from build123d import *

# Parameters (mm, degrees)
CROQUIS1_W              = 8
CROQUIS1_H              = 8
CROQUIS1_R              = 2.5
SALIENTE_EXTRUIR4_DEPTH = 150


with BuildPart() as part:
    # Croquis1 → Saliente-Extruir4 (new body)
    with BuildSketch(Plane.XY):
        with BuildLine():
            Line((-3, 8.7), (-3, 10))
            Line((-3, 10), (-9, 10))
            ThreePointArc((-9, 10), (-9.707106781, 9.707106781), (-10, 9))
            Line((-10, 9), (-10, 3))
            Line((-10, 3), (-8.7, 3))
            Line((-8.7, 3), (-8.7, 6))
            Line((-8.7, 6), (-4, 3.25))
            Line((-4, 3.25), (-4, 4))
            Line((-4, 4), (-3.25, 4))
            Line((-3.25, 4), (-6, 8.7))
            Line((-6, 8.7), (-3, 8.7))
        make_face()
        with BuildLine():
            Line((9, 10), (3, 10))
            Line((3, 10), (3, 8.7))
            Line((3, 8.7), (6, 8.7))
            Line((6, 8.7), (3.25, 4))
            Line((3.25, 4), (4, 4))
            Line((4, 4), (4, 3.25))
            Line((4, 3.25), (8.7, 6))
            Line((8.7, 6), (8.7, 3))
            Line((8.7, 3), (10, 3))
            Line((10, 3), (10, 9))
            ThreePointArc((10, 9), (9.707106781, 9.707106781), (9, 10))
        make_face()
        with BuildLine():
            Line((10, -9), (10, -3))
            Line((10, -3), (8.7, -3))
            Line((8.7, -3), (8.7, -6))
            Line((8.7, -6), (4, -3.25))
            Line((4, -3.25), (4, -4))
            Line((4, -4), (3.25, -4))
            Line((3.25, -4), (6.25, -8.7))
            Line((6.25, -8.7), (3, -8.7))
            Line((3, -8.7), (3, -10))
            Line((3, -10), (9, -10))
            ThreePointArc((9, -10), (9.707106781, -9.707106781), (10, -9))
        make_face()
        with BuildLine():
            Line((-8.7, -3), (-10, -3))
            Line((-10, -3), (-10, -9))
            ThreePointArc((-10, -9), (-9.707106781, -9.707106781), (-9, -10))
            Line((-9, -10), (-3, -10))
            Line((-3, -10), (-3, -8.7))
            Line((-3, -8.7), (-5.75, -8.7))
            Line((-5.75, -8.7), (-3.25, -4))
            Line((-3.25, -4), (-4, -4))
            Line((-4, -4), (-4, -3.25))
            Line((-4, -3.25), (-8.7, -6))
            Line((-8.7, -6), (-8.7, -3))
        make_face()
        Rectangle(CROQUIS1_W, CROQUIS1_H)
        Circle(CROQUIS1_R, mode=Mode.SUBTRACT)
    extrude(amount=SALIENTE_EXTRUIR4_DEPTH)


solid = part.part
Work out the finished part from the listing and answer in its coordinate system (mm). A direction names the side the tool comes from. Round coordinates to 2 decimals unless told otherwise and drop trailing zeros. Write each loop counter-clockwise with the first axis right and the second up, starting at its lowest first coordinate (ties: lowest second). Pieces come first, ordered by that corner, then holes.
1) A cutting plane is placed at A-A (x = 0). Give the vertices of the cut face in (y, z), plus the area to 3 significant figures.
2) The mould has two halves that part along Y. Classify faces 1 (the flat face through (10, 6, 74)), 2 (the flat face through (-6, 10, 74)), 3 (the flat face through (-4.518, -6.383, 73.95)): pulls with the +Y half, pulls with the -Y half, needs draft (parallel to the pull), parting line crosses it, or undercut.
3) Given pin 1 Ø5 at (x, z) = (-1.5, 83) entering from +Y; pin 2 Ø1.5 at (x, y) = (5.5, 0) entering from -Z; pin 3 Ø0.7 at (y, z) = (9.5, 53) entering from -X, each flat-ended and moving along its own axis, determine where each tip first touches the part or whether it passes through.
4) Straight lines are drawn through the part: line 1 (Y direction, x = 0, z = 74); line 2 (X direction, y = -5.25, z = 131.5); line 3 (Y direction, x = -1, z = 88). For each, find the intervals that lie inside material, in ascending order.
5) A tool of negligible diameter and unlimited length cuts with its end or side. For faces 4 (the flat face through (2, 2, 0)), 5 (the flat face through (4.644, 6.383, 73.95)), from which of +Z, -Z, +X, -X, +Y, -Y can it reach the whole face along a straight path? Write none if from no direction.
Completed:
1. outline: (-4, 0) - (-2.5, 0) - (-2.5, 150) - (-4, 150) - close; (2.5, 0) - (4, 0) - (4, 150) - (2.5, 150) - close
1. area: 450 mm2
2. face 1: needs draft
2. face 2: pulls with the +Y half
2. face 3: undercut
3. pin 1: stops at y = 10
3. pin 2: passes through
3. pin 3: stops at x = -9.99
4. line 1: y = -4 to -2.5, 2.5 to 4
4. line 2: x = -10 to -8.7, -7.42 to -3.91, 4.05 to 7.42, 8.7 to 10
4. line 3: y = -4 to -2.29, 2.29 to 4
5. face 4: -Z, +X, -X, +Y, -Y
5. face 5: +Z, -Z
